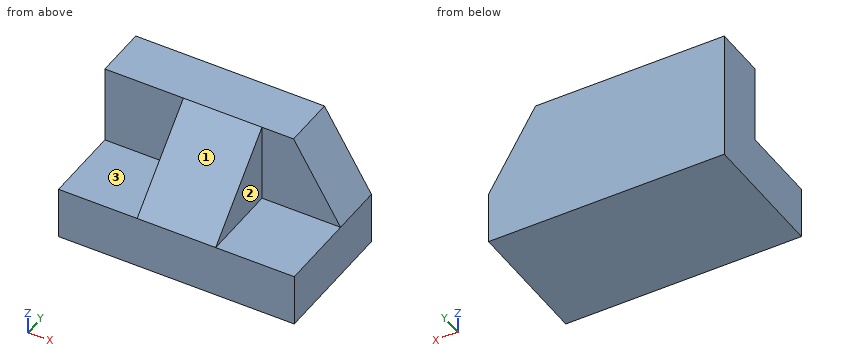
from build123d import *

# Parameters (mm, degrees)
F0_W     = 31.75
F0_H     = 31.75
F1_DEPTH = 57.15
F2_W     = 19.05
F2_H     = 19.05
F3_DEPTH = 19.05
F4_W     = 19.05
F4_H     = 19.05
F5_DEPTH = 19.05
F7_DEPTH = 25.4
F9_DEPTH = 25.4


with BuildPart() as f1:
    # F0 (on Right) → F1 (new body)
    with BuildSketch(Plane.YZ):
        with Locations((-15.875, 15.875)):
            Rectangle(F0_W, F0_H)
    extrude(amount=F1_DEPTH)

    # F2 (on face) → F3 (cut)
    with BuildSketch(Plane(origin=(0, 0, 0), x_dir=(0, -1, 0), z_dir=(-1, 0, 0))):
        with Locations((22.225, 22.225)):
            Rectangle(F2_W, F2_H)
    extrude(amount=-F3_DEPTH, mode=Mode.SUBTRACT)

    # F4 (on face) → F5 (cut)
    with BuildSketch(Plane.YZ.offset(57.15)):
        with Locations((-22.225, 22.225)):
            Rectangle(F4_W, F4_H)
    extrude(amount=-F5_DEPTH, mode=Mode.SUBTRACT)

    # F6 (on face) → F7 (cut)
    with BuildSketch(Plane.XZ.offset(12.7)):
        Polygon((45.753013, 31.75), (57.15, 12.7), (57.15, 31.75), align=None)
    extrude(amount=-F7_DEPTH, mode=Mode.SUBTRACT)

    # F8 (on face) → F9 (cut)
    with BuildSketch(Plane(origin=(19.05, 0, 0), x_dir=(0, -1, 0), z_dir=(-1, 0, 0))):
        Polygon((12.7, 31.75), (31.75, 12.7), (31.75, 31.75), align=None)
    extrude(amount=-F9_DEPTH, mode=Mode.SUBTRACT)


solid = f1.part
Can you work these out from the model? Positions are in its coordinate system, mm. Face numbers are marked on the shaded views. A direction names the side the tool comes from. Give positions to 0.01 mm unless a question says otherwise; leave off trailing zeros. Order: outer loops, then holes, each group sorted by start corner. A loop starts at its lowest first (then second) coordinate and runs counter-clockwise, first axis right, second up. Notation, with made-up numbers: M 63.25,3 L 81.25,3 A27 cw 81.25,26 Z; hole C 11.5,31 d3. An arc over 180 degrees is marked long. One line per question, with ' | ' between items.
Item 1: Suppose I cut it at D-D, the plane x = 8.5. Write out the boundary of the cut face in (y, z), then the cut area to 3 significant figures.
Answer block:
outline: M -31.75,0 L 0,0 L 0,31.75 L -12.7,31.75 L -12.7,12.7 L -31.75,12.7 Z | area: 645 mm2
Item 2: Please list where these lines run through material, in increasing order: L1, parallel to Z at x = 51.5, y = -20.5; L2, parallel to Y at x = 38.5, z = 21.5; L3, parallel to X at y = -26.5, z = 15.
Answer block:
L1: z = 0 to 12.7 | L2: y = -12.7 to 0 | L3: x = 19.05 to 38.1
Item 3: I'm going to push flat-ended pins straight in: pin 1 Ø9.5 at (x, z) = (49, 22.5) entering from -Y; pin 2 Ø4 at (x, y) = (23.5, -6.5) entering from -Z; pin 3 Ø15 at (y, z) = (-24, 23.5) entering from +X; pin 4 Ø9.5 at (x, y) = (8, -22) entering from +Z. Where does each tip first touch, or does it pass through?
Answer block:
pin 1: stops at y = -12.7 | pin 2: stops at z = 0 | pin 3: stops at x = 38.1 | pin 4: stops at z = 12.7
Item 4: For the marked faces 1, 2 and 3, which set-ups out of +Z, -Z, +X, -X, +Y, -Y let a thin tool reach every point of the face, with its end or its side?
Answer block:
face 1: +Z, +X, -X, -Y | face 2: +Z, +X, -Y | face 3: +Z, -X, -Y
Item 5: Suppose I cut it at A-A, the plane y = -29. Write out the boundary of the cut face in (x, z), then the cut area to 3 significant figures.
Answer block:
outline: M 0,0 L 57.15,0 L 57.15,12.7 L 38.1,12.7 L 38.1,15.45 L 19.05,15.45 L 19.05,12.7 L 0,12.7 Z | area: 778 mm2
Item 6: Suppose I cut it at C-C, the plane z = 29. Write out the boundary of the cut face in (x, y), then the cut area to 3 significant figures.
Answer block:
outline: M 0,-12.7 L 19.05,-12.7 L 19.05,-15.45 L 38.1,-15.45 L 38.1,-12.7 L 47.4,-12.7 L 47.4,0 L 0,0 Z | area: 654 mm2
Item 7: Suppose I cut it at B-B, the plane x = 32. Write out the boundary of the cut face in (y, z).
Answer block:
outline: M -31.75,0 L 0,0 L 0,31.75 L -12.7,31.75 L -31.75,12.7 Z
